The drawing under review shows one solid part. Ordinate dimensions are in mm from its lowest x, y, z. Coordinates: 2 decimals unless noted, no trailing zeros. Order: outer loops, then holes, each group sorted by start corner. A loop starts at its lowest first (then second) coordinate and runs counter-clockwise, first axis right, second up.
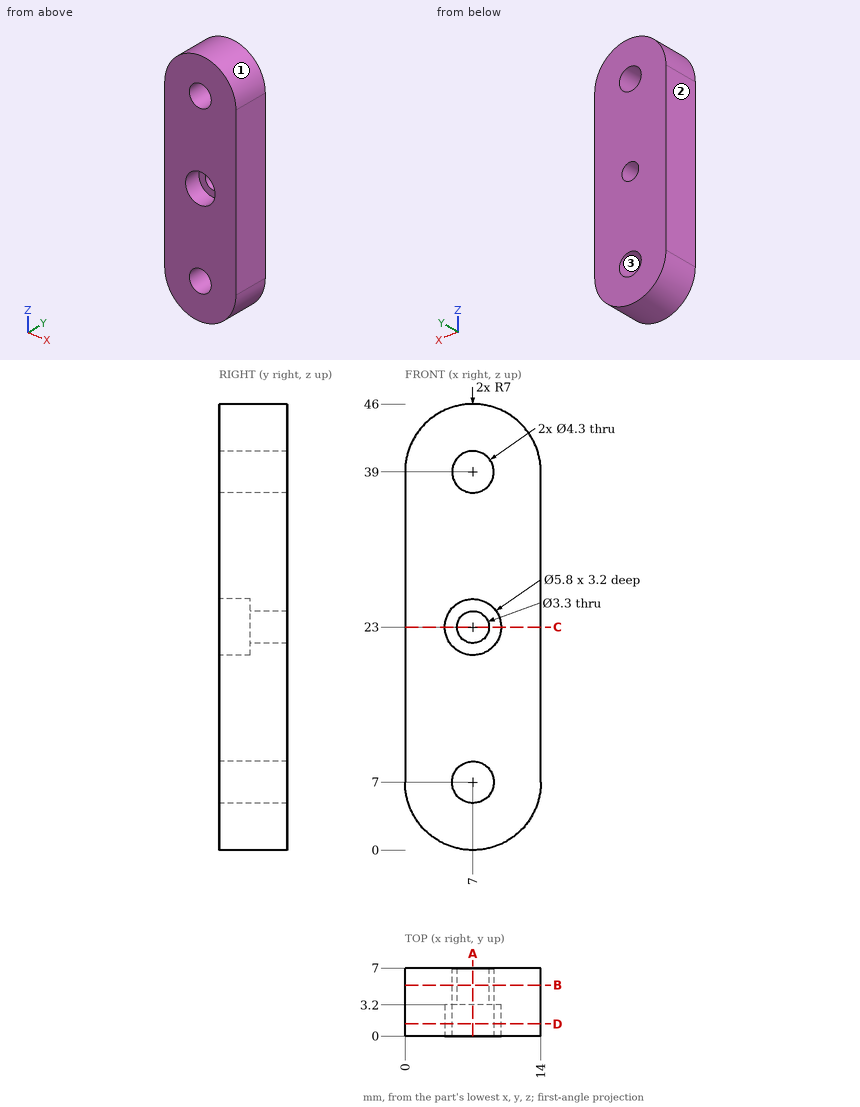
(1) Wall thickness on probe 1 along Z at (x, y) = (7, 2.45); probe 2 along Z at (x, y) = (7, 5.35); probe 3 along X at (y, z) = (1.5, 39): over which ranges is each line inside the solid? List them lowest first.
A:
probe 1: z = 0 to 4.85, 9.15 to 20.1, 25.9 to 36.85, 41.15 to 46
probe 2: z = 0 to 4.85, 9.15 to 21.35, 24.65 to 36.85, 41.15 to 46
probe 3: x = 0 to 4.85, 9.15 to 14
(2) We need section A-A, the plane x = 7. Write out the cut boundary in (y, z).
A:
outline: (0, 0) - (7, 0) - (7, 4.85) - (0, 4.85) - close; (0, 9.15) - (7, 9.15) - (7, 21.35) - (3.2, 21.35) - (3.2, 20.1) - (0, 20.1) - close; (0, 25.9) - (3.2, 25.9) - (3.2, 24.65) - (7, 24.65) - (7, 36.85) - (0, 36.85) - close; (0, 41.15) - (7, 41.15) - (7, 46) - (0, 46) - close
(3) We need section D-D, the plane y = 1.25. Write out the cut boundary in (x, z), and give its area (3 significant figures).
A:
outline: (0, 7) arc R7 ccw to (14, 7) - (14, 39) arc R7 ccw to (0, 39) - close; hole circle Ø5.8 at (7, 23); hole circle Ø4.3 at (7, 7); hole circle Ø4.3 at (7, 39)
area: 546 mm2
(4) We need section C-C, the plane z = 23. Write out the cut boundary in (x, y).
A:
outline: (0, 0) - (4.1, 0) - (4.1, 3.2) - (5.35, 3.2) - (5.35, 7) - (0, 7) - close; (8.65, 3.2) - (9.9, 3.2) - (9.9, 0) - (14, 0) - (14, 7) - (8.65, 7) - close
(5) For pin 1 Ø6.5 at (x, z) = (7, 23) entering from -Y; pin 2 Ø5.5 at (x, z) = (7, 23) entering from -Y; pin 3 Ø2 at (x, y) = (12.5, 5.5) entering from -Z; pin 4 Ø3 at (x, y) = (3.5, 6.5) entering from +Z, all flat-tipped, find the tip position at first contact; note any pin that passes through.
A:
pin 1: stops at y = 0
pin 2: stops at y = 3.2
pin 3: stops at z = 1.64
pin 4: stops at z = 45.71
(6) We need section B-B, the plane y = 5.25. Write out the cut boundary in (x, z).
A:
outline: (0, 7) arc R7 ccw to (14, 7) - (14, 39) arc R7 ccw to (0, 39) - close; hole circle Ø4.3 at (7, 7); hole circle Ø4.3 at (7, 39); hole circle Ø3.3 at (7, 23)
(7) Draft analysis for pull direction X (two halves, no side actions). For the marked faces 1, 2 and 3, state which applies: released by +X, released by -X, zero draft, split by the parting line, or undercut.
A:
face 1: split by the parting line
face 2: released by -X
face 3: undercut
